from build123d import *

# Parameters (mm, degrees)
EXTRUDE_1_DEPTH = 40
SKETCH_3_W      = 4
SKETCH_3_H      = 32
EXTRUDE_2_DEPTH = 160
EXTRUDE_3_DEPTH = 40


with BuildPart() as part:
    # 草图2 → 凸台-拉伸1 (new body)
    with BuildSketch(Plane(origin=(0, 0, 0), x_dir=(1, 0, 0), z_dir=(0, 1, 0))):
        with BuildLine():
            Line((-40, -80), (40, -80))
            ThreePointArc((40, -80), (96.568542495, -56.568542495), (120, 0))
            Line((120, 0), (120, 16))
            Line((120, 16), (124, 16))
            Line((124, 16), (124, -16))
            Line((124, -16), (122.462112512, -16))
            ThreePointArc((122.462112512, -16), (93.441556864, -64.807406984), (40, -84))
            Line((40, -84), (-40, -84))
            ThreePointArc((-40, -84), (-93.441556864, -64.807406984), (-122.462112512, -16))
            Line((-122.462112512, -16), (-124, -16))
            Line((-124, -16), (-124, 16))
            Line((-124, 16), (-120, 16))
            Line((-120, 16), (-120, 0))
            ThreePointArc((-120, 0), (-96.568542495, -56.568542495), (-40, -80))
        make_face()
    extrude(amount=EXTRUDE_1_DEPTH)

    # 草图3 → 凸台-拉伸2 (add)
    with BuildSketch(Plane.XZ):
        with Locations((-122, 0)):
            Rectangle(SKETCH_3_W, SKETCH_3_H)
        with Locations((122, 0)):
            Rectangle(SKETCH_3_W, SKETCH_3_H)
    extrude(amount=EXTRUDE_2_DEPTH)

    # 草图5 → 凸台-拉伸3 (add)
    with BuildSketch(Plane(origin=(0, 40, 0), x_dir=(1, 0, 0), z_dir=(0, 1, 0))):
        Polygon((-40, -84), (-78, -84), (-78, -74.913283201), (-55.5334574, -80.946187921), (52.897278528, -80.946187921), (78, -72.607731722), (78, -84), (40, -84), align=None)
    extrude(amount=-EXTRUDE_3_DEPTH)


solid = part.part
Can you work these out from the model? Positions are in its coordinate system, mm. A direction names the side the tool comes from. Give positions to 0.01 mm unless a question says otherwise; leave off trailing zeros. Order: outer loops, then holes, each group sorted by start corner. A loop starts at its lowest first (then second) coordinate and runs counter-clockwise, first axis right, second up. Notation, with made-up numbers: M 1.25,-19 L 45.25,-19 A17 cw 45.25,9 Z; hole C 35,7 d5. An arc over 180 degrees is marked long. Use a Markdown table: item, result. Add a question column.
Item 1: If I drill on L1, parallel to X at y = -147.5, z = 3; L2, parallel to Y at x = 108, z = 48; L3, parallel to X at y = 6, z = 44, over which ranges is the centre line in solid material (lowest first)? Write a range as [from, to].
Item 2: Will these pins go through, and if not, where does the flat tip stop? pin 1 (8 mm diameter, centred on y = 17.5, z = 64, fed in from +X); pin 2 (12 mm diameter, centred on y = 1.5, z = 51, fed in from -X); pin 3 (2.5 mm diameter, centred on y = 14.5, z = 80.5, fed in from -X); pin 4 (10 mm diameter, centred on y = -55.5, z = 22.5, fed in from +X).
Item 3: Suppose I cut it at A-A (z = 40). List the corners of the cut face in (x, y) for me, then the cut area to 3 significant figures.
Item 4: Suppose I cut it at B-B (y = -129.5). List the corners of the cut face in (x, z) for me.
Item 5: We'd pull the mould along X, two halves only. Please class faces 6 (the flat face through (120, -59, 0)), 7 (the flat face through (-1, 20, 84)), 8 (the cylindrical face through (-106.725, 19.72, 51.028)): +X half, -X half, draft (parallel to the pull), parting line (faces both ways), or undercut.
Item 6: For faces 1 (the flat face through (78, 20, 79)), 2 (the flat face through (124, -61, 0)), 3 (the flat face through (-120, -59, 0)), 4 (the flat face through (-1, 20, 80)), 5 (the flat face through (-78, 20, 80)), which set-ups out of +Z, -Z, +X, -X, +Y, -Y let a thin tool reach every point of the face, with its end or its side?
Item 7: Suppose I cut it at D-D (x = 94). List the corners of the cut face in (y, z) for me, then the cut area to 3 significant figures.
Item 8: Suppose I cut it at C-C (x = -10). List the corners of the cut face in (y, z) for me.
Answer sheet:
| question | item | result |
|---|---|---|
| 1 | L1 | x = [-124, -120], [120, 124] |
| 1 | L2 | y = [0, 40] |
| 1 | L3 | x = [-111.55, -106.81], [106.81, 111.55] |
| 2 | pin 1 | stops at x = 98.79 |
| 2 | pin 2 | stops at x = -110.93 |
| 2 | pin 3 | stops at x = -78 |
| 2 | pin 4 | passes through |
| 3 | outline | M -113.86,0 L -109.28,0 L -109.28,40 L -113.86,40 Z; M 109.28,0 L 113.86,0 L 113.86,40 L 109.28,40 Z |
| 3 | area | 367 mm² |
| 4 | outline | M -124,-16 L -120,-16 L -120,16 L -124,16 Z; M 120,-16 L 124,-16 L 124,16 L 120,16 Z |
| 5 | face 6 | undercut |
| 5 | face 7 | draft |
| 5 | face 8 | -X half |
| 6 | face 1 | +Z, +X, +Y, -Y |
| 6 | face 2 | +Z, -Z, +X, +Y, -Y |
| 6 | face 3 | -Z, -Y |
| 6 | face 4 | -Z, +Y, -Y |
| 6 | face 5 | +Z, -X, +Y, -Y |
| 7 | outline | M 0,59.03 L 40,59.03 L 40,64.34 L 0,64.34 Z |
| 7 | area | 213 mm² |
| 8 | outline | M 0,80 L 40,80 L 40,84 L 0,84 Z |
